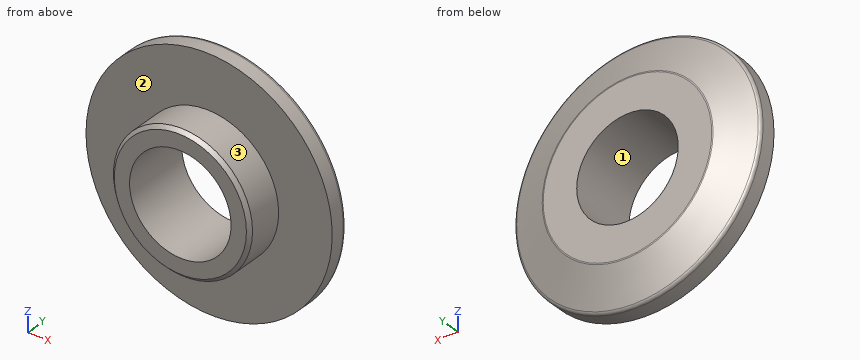
from build123d import *

# Parameters (mm, degrees)
SKETCH1_R           = 22.479
SKETCH1_R_2         = 9.271
BOSS_EXTRUDE1_DEPTH = 12.446
SKETCH2_R           = 22.479
SKETCH2_R_2         = 12.7
CUT_EXTRUDE1_DEPTH  = 6.858
CHAMFER1_SIZE       = 2.54
CHAMFER1_SIZE2      = 6.978592645
CHAMFER2_SIZE       = 0.635
FILLET1_R           = 0.635


with BuildPart() as part:
    # Sketch1 → Boss-Extrude1 (new body)
    with BuildSketch(Plane(origin=(0, 0, 0), x_dir=(1, 0, 0), z_dir=(0, 1, 0))):
        Circle(SKETCH1_R)
        Circle(SKETCH1_R_2, mode=Mode.SUBTRACT)
    extrude(amount=BOSS_EXTRUDE1_DEPTH)

    # Sketch2 → Cut-Extrude1 (cut)
    with BuildSketch(Plane.XZ):
        Circle(SKETCH2_R)
        Circle(SKETCH2_R_2, mode=Mode.SUBTRACT)
    extrude(amount=-CUT_EXTRUDE1_DEPTH, mode=Mode.SUBTRACT)

    # Chamfer1
    chamfer1_edges = [part.edges().sort_by_distance(p)[0] for p in [
        (-22.479, 12.446, 0),
    ]]
    chamfer1_side = [part.faces().sort_by_distance(p)[0] for p in [
        (-22.479, 9.652, 0),
    ]]
    chamfer(chamfer1_edges, length=CHAMFER1_SIZE, length2=CHAMFER1_SIZE2, reference=chamfer1_side[0])

    # Chamfer2
    chamfer2_edges = [part.edges().sort_by_distance(p)[0] for p in [
        (-12.7, 0, 0),
    ]]
    chamfer(chamfer2_edges, length=CHAMFER2_SIZE)

    # Fillet1
    fillet1_edges = [part.edges().sort_by_distance(p)[0] for p in [
        (-15.500407355, 12.446, 0),
        (-22.479, 9.906, 0),
    ]]
    fillet(fillet1_edges, radius=FILLET1_R)


solid = part.part
Work out the finished part from the listing and answer in its coordinate system (mm). Face numbers are marked on the shaded views. Give positions to 0.01 mm unless a question says otherwise; leave off trailing zeros. Order: outer loops, then holes, each group sorted by start corner. A loop starts at its lowest first (then second) coordinate and runs counter-clockwise, first axis right, second up. Notation, with made-up numbers: (5, 87) -> (59, 87) arc R32 cw to (59, 118) -> close; hole circle Ø10 at (61, -0.75). An arc over 180 degrees is marked (long way). One line per item, written item: value.
Item 1: Find section A-A, the plane y = 8.75. Give the vertices of the cut face in (x, z).
Answer sheet:
outline: circle Ø44.96 at (0, 0); hole circle Ø18.54 at (0, 0)
Item 2: Straight lines are drawn through the part: probe 1 along Z at (x, y) = (0, 4.5); probe 2 along X at (y, z) = (8, 0). For each, find the intervals that lie inside material, in ascending order.
Answer sheet:
probe 1: -12.7 to -9.27, 9.27 to 12.7
probe 2: -22.48 to -9.27, 9.27 to 22.48
Item 3: Determine the mould class of the marked faces 1, 2 and 3 for opening direction Z: released by +Z, released by -Z, zero draft, split by the parting line, or undercut.
Answer sheet:
face 1: undercut
face 2: zero draft
face 3: split by the parting line
Item 4: Flat-ended cylindrical pins translate along their axes: P1, Ø10, axis at x = -15, z = 16, coming from the +Y side; P2, Ø4, axis at x = 13, z = 12.5, coming from the -Y side; P3, Ø1, axis at y = 2.5, z = 6.5, coming from the +X side. Find the tip coordinate at first contact, or state that the pin passes through.
Answer sheet:
P1: y = 11.93
P2: y = 6.86
P3: x = 11.19
